```python
from build123d import *

# Parameters (mm, degrees)
SKETCH_1_W      = 50
SKETCH_1_H      = 22
SKETCH_1_R      = 1.5
EXTRUDE_1_DEPTH = 1
OTHER_START     = -10.142952565
OTHER_1_DEPTH   = 22
OTHER_1_2_DEPTH = 22
FILLET_1_R      = 2


# Read off the part's stored shape, not the designer's step: Нарисованный сгиб1
with BuildPart() as part:
    # Sketch 1 → Бобышка-Вытянуть1 (new body)
    with BuildSketch(Plane(origin=(0, 0, 0), x_dir=(1, 0, 0), z_dir=(0, 1, 0))):
        with Locations((0, -0.857047435)):
            Rectangle(SKETCH_1_W, SKETCH_1_H)
        with Locations(Location((-18, -0.857047435, 0), (0, 0, 270))):
            Circle(SKETCH_1_R, mode=Mode.SUBTRACT)
        with BuildLine():
            ThreePointArc((-5.514009268, -2.575584316), (-5.396296831, -0.857047435), (-5.514009268, 0.861489446))
            ThreePointArc((-5.514009268, 0.861489446), (-7.204527613, 2.142952565), (-8.485990732, 0.45243422))
            ThreePointArc((-8.485990732, 0.45243422), (-8.396296831, -0.857047435), (-8.485990732, -2.16652909))
            ThreePointArc((-8.485990732, -2.16652909), (-7.204527613, -3.857047435), (-5.514009268, -2.575584316))
        make_face(mode=Mode.SUBTRACT)
    extrude(amount=EXTRUDE_1_DEPTH)

    # Other 1 outline → Other 1 (cut)
    with BuildSketch(Plane.XY.offset(OTHER_START)):
        with BuildLine():
            Line((25, 1), (0.628815399, 1))
            ThreePointArc((0.628815399, 1), (0.08062724, 0.275255129), (-0.785398163, 0))
            Line((-0.785398163, 0), (25, 0))
            Line((25, 0), (25, 1))
        make_face()
    extrude(amount=OTHER_1_DEPTH, mode=Mode.SUBTRACT)

    # Other 1 2 outline → Other 1 2 (add)
    with BuildSketch(Plane.XY.offset(OTHER_START)):
        with BuildLine():
            Line((0.714601837, 1.5), (0.714601837, 25.714601837))
            Line((0.714601837, 25.714601837), (-0.285398163, 25.714601837))
            Line((-0.285398163, 25.714601837), (-0.285398163, 1.5))
            ThreePointArc((-0.285398163, 1.5), (-0.431844772, 1.146446609), (-0.785398163, 1))
            Line((-0.785398163, 1), (0.628815399, 1))
            ThreePointArc((0.628815399, 1), (0.692999676, 1.246347032), (0.714601837, 1.5))
        make_face()
    extrude(amount=OTHER_1_2_DEPTH)

    # Скругление1
    fillet_1_edges = [part.edges().sort_by_distance(p)[0] for p in [
        (0.214601837, 25.714601837, -10.142952565),
        (0.214601837, 25.714601837, 11.857047435),
        (-25, 0.5, 11.857047435),
        (-25, 0.5, -10.142952565),
    ]]
    fillet(fillet_1_edges, radius=FILLET_1_R)


solid = part.part
```
The listing builds one solid part. Answer for the finished solid, in the listing's coordinates (mm). A direction names the side the tool comes from. Give positions to 0.01 mm unless a question says otherwise; leave off trailing zeros. Write each loop counter-clockwise with the first axis right and the second up, starting at its lowest first coordinate (ties: lowest second). Pieces come first, ordered by that corner, then holes. Notation, with made-up numbers: M 68,54 L 119,54 A15 cw 119,63 Z; hole C 59,76.25 d8. An arc over 180 degrees is marked long. Write each question's results on one line, items separated by ' | '.
Q1. Section A-A, the plane x = -7 is taken. Write down the section's boundary in (y, z).
Output values:
outline: M 0,-10.14 L 1,-10.14 L 1,-2.16 L 0,-2.16 Z; M 0,3.87 L 1,3.87 L 1,11.86 L 0,11.86 Z
Q2. Section B-B, the plane z = 1.5 is taken. Write down the section's boundary in (x, y).
Output values:
outline: M -25,0 L -19.36,0 L -19.36,1 L -25,1 Z; M -16.64,0 L -8.42,0 L -8.42,1 L -16.64,1 Z; M -5.41,0 L -0.79,0 A1.5 ccw 0.71,1.5 L 0.71,25.71 L -0.29,25.71 L -0.29,1.5 A0.5 cw -0.79,1 L -5.41,1 Z
Q3. Section D-D, the plane z = 6.5 is taken. Write down the section's boundary in (x, y), then the cut area to 3 significant figures.
Output values:
outline: M -25,0 L -0.79,0 A1.5 ccw 0.71,1.5 L 0.71,25.71 L -0.29,25.71 L -0.29,1.5 A0.5 cw -0.79,1 L -25,1 Z | area: 50.0 mm2
Q4. Consider L1, parallel to X at y = 13.25, z = -8.5; L2, parallel to Y at x = -13.75, z = 1.5; L3, parallel to Y at x = -0.25, z = -2.5. Determine where each line is inside the solid, lowest interval first. Write a range as from..to.
Output values:
L1: -0.29..0.71 | L2: 0..1 | L3: 0.1..25.71
Q5. For a pull along X with two mould halves and no side action, classify faces 1 (the cylindrical face through (-7.172, 0.493, -2.147)), 2 (the cylindrical face through (-16.735, 0.493, 1.663)), 3 (the flat face through (-13, 1, 1)), 4 (the flat face through (-0.285, 14, 1)) as released by +X, released by -X, zero draft, split by the parting line, or undercut.
Output values:
face 1: undercut | face 2: undercut | face 3: zero draft | face 4: released by -X
Q6. Flat-ended cylindrical pins translate along their axes: P1, Ø8, axis at x = -16, z = -0.5, coming from the +Y side; P2, Ø5, axis at y = 4, z = -2.5, coming from the -X side. Find the tip coordinate at first contact, or state that the pin passes through.
Output values:
P1: y = 1 | P2: x = -0.29
Q7. A tool of negligible diameter and unlimited length cuts with its end or side. For faces 5 (the cylindrical face through (-8.396, 0.493, 0.839)), 6 (the flat face through (-25, 0.5, 1)), from which of +Z, -Z, +X, -X, +Y, -Y can it reach the whole face along a straight path? Write none if from no direction.
Output values:
face 5: +Y, -Y | face 6: +Z, -Z, -X, +Y, -Y
Q8. Section C-C, the plane x = -18 is taken. Write down the section's boundary in (y, z), then the cut area to 3 significant figures.
Output values:
outline: M 0,-10.14 L 1,-10.14 L 1,-0.64 L 0,-0.64 Z; M 0,2.36 L 1,2.36 L 1,11.86 L 0,11.86 Z | area: 19.0 mm2
